Verification items for the finished model (mm, model axes). A direction names the side the tool comes from. Coordinates: 2 decimals unless noted, no trailing zeros. Order: outer loops, then holes, each group sorted by start corner. A loop starts at its lowest first (then second) coordinate and runs counter-clockwise, first axis right, second up. Notation, with made-up numbers: M 23,-6.5 L 63,-6.5 A21 ccw 63,9.5 Z; hole C 23,75.25 d3. An arc over 180 degrees is marked long. Answer as a JSON object with one key per item and string values. Group by question number.
(1) Gauge pin test, flat ends, axial feed: pin 1 Ø1 at (x, y) = (2, 100.5) entering from -Z; pin 2 Ø1.5 at (x, y) = (2, 25) entering from +Z. Record the tip position at first contact, or that the pin passes through.
(2) Cross-section at D-D (z = 21.5). Enter the section's corners in (x, y), plus the area to 3 significant figures.
(3) Cross-section at B-B (z = 13). Enter the section's corners in (x, y), plus the area to 3 significant figures.
(4) Access from +Z, -Z, +X, -X, +Y, -Y to the whole of each face (thin tool, end or side, straight path). Record for faces 1 (the face through (2.465, 16.368, 11.035)), 2 (the face through (2.465, 102.856, 15.252)), 3 (the face through (2.46, 18.89, 4.51)).
(5) Cross-section at C-C (x = 1.7). Enter the section's corners in (y, z).
(6) Mould release check, pull along Z, two halves, no side actions. Record for faces 4 (the face through (5, 77, 6)), 5 (the face through (2.465, 54.637, 0.756)), 6 (the face through (2.5, 113.8, 18.6)), 7 (the face through (2.46, 59.56, 6.89)): released by +Z, released by -Z, zero draft, split by the parting line, or undercut.
(7) Cross-section at A-A (y = 94.5). Enter the section's corners in (x, z).
(8) Material ranges on line 1 (Z direction, x = 0.55, y = 29.5); line 2 (Z direction, x = 2.75, y = 100.5); line 3 (Z direction, x = 3.55, y = 56.5), recorded low to high.
from build123d import *

# Parameters (mm, degrees)
F0_R     = 2.5
F1_DEPTH = 5


# Not quite as in the source:
# - a feature names something its author has since deleted; it is built from what else it names


with BuildPart() as f1:
    # F0 (on Right) → F1 (new body)
    with BuildSketch(Plane.YZ):
        with BuildLine():
            ThreePointArc((118.6011307413, 10.3511984734), (119.6029410321, 10.9159653279), (119.9999999073, 11.9952844227))
            ThreePointArc((119.9999999073, 11.9952844227), (119.8357295493, 18.2767765127), (119.3428752162, 24.5410579746))
            ThreePointArc((119.3428752162, 24.5410579746), (118.5020303548, 25.9696085801), (116.872434029, 26.2732411356))
            Line((116.872434029, 26.2732411356), (78.344444671, 16.7187866332))
            ThreePointArc((78.344444671, 16.7187866332), (50.4120849121, 12.3407543123), (22.1844688263, 10.7327808001))
            ThreePointArc((22.1844688263, 10.7327808001), (22.4292060309, 10.7620820299), (22.6716738588, 10.8064014821))
            Line((22.6716738588, 10.8064014821), (9.8850433167, 11.2693933781))
            Line((9.8850433167, 11.2693933781), (16.5052597895, 5.9341389572))
            ThreePointArc((16.5052597895, 5.9341389572), (18.9230306979, 4.4941821172), (21.6462541623, 3.7848543869))
            Line((21.6462541623, 3.7848543869), (43.8305606526, 1.2529498543))
            ThreePointArc((43.8305606526, 1.2529498543), (54.7908574561, 0.7592543704), (65.7156304083, 1.7697874952))
            Line((65.7156304083, 1.7697874952), (118.6011307413, 10.3511984734))
        make_face()
        with BuildLine():
            ThreePointArc((41.0425990366, 10.096905354), (44.3135999527, 6.3287058646), (40.4926591764, 3.1194713813))
            Line((40.4926591764, 3.1194713813), (21.6135530725, 4.9170973917))
            ThreePointArc((21.6135530725, 4.9170973917), (21.5948304706, 4.9188091028), (21.5761212705, 4.9206615636))
            ThreePointArc((21.5761212705, 4.9206615636), (19.3333513171, 7.4955245428), (21.7516674536, 9.9062678907))
            ThreePointArc((21.7516674536, 9.9062678907), (21.8070986498, 9.9074304985), (21.8625419965, 9.9073635786))
            Line((21.8625419965, 9.9073635786), (40.5372507264, 10.0919113847))
            ThreePointArc((40.5372507264, 10.0919113847), (40.7898346274, 10.1035413352), (41.0425990366, 10.096905354))
        make_face(mode=Mode.SUBTRACT)
        with Locations((50.3031872213, 6.8563437089)):
            Circle(F0_R, mode=Mode.SUBTRACT)
        with BuildLine():
            ThreePointArc((97.4222943066, 19.082035474), (102.8677433707, 15.1465744396), (98.3342272396, 10.1879455412))
            Line((98.3342272396, 10.1879455412), (64.1951699406, 3.8271960831))
            ThreePointArc((64.1951699406, 3.8271960831), (59.5398910648, 6.9765078631), (62.6292671904, 11.6717758272))
            Line((62.6292671904, 11.6717758272), (97.4222943066, 19.082035474))
        make_face(mode=Mode.SUBTRACT)
        with Locations((111.4225909114, 17.8264938295)):
            Circle(F0_R, mode=Mode.SUBTRACT)
    extrude(amount=F1_DEPTH)


solid = f1.part
Taken from the geometry:
{
 "1": {"pin 1": "stops at z = 7.33", "pin 2": "stops at z = 10.78"},
 "2": {"outline": "M 0,97.62 L 5,97.62 L 5,119.62 L 0,119.62 Z", "area": "110 mm²"},
 "3": {"outline": "M 0,56.06 L 5,56.06 L 5,68.87 L 0,68.87 Z; M 0,102.56 L 5,102.56 L 5,120 L 0,120 Z", "area": "151 mm²"},
 "4": {"face 1": "+Z, +X, -X", "face 2": "+X, -X", "face 3": "-Z, +X, -X, -Y"},
 "5": {"outline": "M 9.89,11.27 L 16.51,5.93 A10 ccw 21.65,3.78 L 43.83,1.25 A80 ccw 65.72,1.77 L 118.6,10.35 A1.67 ccw 120,12 A120 ccw 119.34,24.54 A2 ccw 116.87,26.27 L 78.34,16.72 A286.95 cw 22.18,10.73 A4 ccw 22.67,10.81 Z; hole M 21.61,4.92 L 40.49,3.12 A3.5 ccw long 40.54,10.09 L 21.86,9.91 A2.5 ccw Z; hole C 50.3,6.86 d5; hole M 62.63,11.67 A4 ccw 64.2,3.83 L 98.33,10.19 A4.5 ccw long 97.42,19.08 Z; hole C 111.42,17.83 d5"},
 "6": {"face 4": "zero draft", "face 5": "released by -Z", "face 6": "undercut", "face 7": "undercut"},
 "7": {"outline": "M 0,6.44 L 5,6.44 L 5,9.47 L 0,9.47 Z; M 0,18.46 L 5,18.46 L 5,20.73 L 0,20.73 Z"},
 "8": {"line 1": "z = 2.89 to 4.17, 9.98 to 10.88", "line 2": "z = 7.41 to 10.71, 18.66 to 22.21", "line 3": "z = 0.82 to 13.06"}
}
